Autodesk Inventor part; units mm, degrees
ref_plane "Work Plane1" through (1.525, 0, 0) normal (0, 0, 1) x (1, 0, 0)
ref_plane "YZ Plane" through (0, 0, 0) normal (1, 0, 0) x (0, 1, 0)
ref_plane "XZ Plane" through (0, 0, 0) normal (0, 1, 0) x (-1, 0, 0)
sketch "Sketch1" plane through (0, 0, 0) normal (0, 0, 1) x (1, 0, 0)
  line L0 (0, 7.1374) -> (0, 4.7625)
  line L1 (50.8, 4.7625) -> (76.2, 4.7625)
  line L2 (76.2, 4.7625) -> (76.2, 0)
  line L3 (76.2, 0) -> (-0.6351, 0)
  line L4 (-16.0021, 0) -> (91.567, 0)
  line L5 (-0.6351, 0) -> (-0.6351, 7.1374)
  line L6 (-0.6351, 7.1374) -> (0, 7.1374)
  line L7 (50.8, 4.7625) -> (39.6747, 4.7625)
  line L8 (39.6747, 4.7625) -> (0, 4.7625)
  line L9 (0, -1.4275) -> (0, 8.5649)
  dimension "d0" = 76.2
  dimension "d1" = 25.4
  dimension "d2" = 9.525
  dimension "d9" = 0.6351
  dimension "d10" = 14.2748
  dimension "d13" = 11.1253
  dimension "d14" = 9.525
revolve "Body" add sketch "Sketch1" angle 360 about axis through (76.2, 0, 0) along (-1, 0, 0)
sketch "Sketch2" plane through (-0.6351, 0, 0) normal (-1, 0, 0) x (0, 0, 1)
  line L0 (0, 8.2416) -> (7.1374, 4.1208)
  line L1 (7.1374, 4.1208) -> (7.1374, -4.1208)
  line L2 (7.1374, -4.1208) -> (0, -8.2416)
  line L3 (0, -8.2416) -> (-7.1374, -4.1208)
  line L4 (-7.1374, -4.1208) -> (-7.1374, 4.1208)
  line L5 (-7.1374, 4.1208) -> (0, 8.2416)
  point P0 (0, 0)
  point P1 (0, 0)
  dimension "d11" = 14.2748
extrude "Head" add sketch "Sketch2" along normal blind 5.5372
sketch "Sketch4" plane through (0, 0, 0) normal (0, 0, 1) x (1, 0, 0)
  line L0 (-6.1723, 7.1374) -> (-6.1723, 8.2416)
  line L1 (-6.1723, 8.2416) -> (-5.5348, 8.2416)
  line L2 (-5.5348, 8.2416) -> (-6.1723, 7.1374)
  line L3 (-7.2797, 0) -> (0.4723, 0)
  line L4 (-0.6351, 8.2416) -> (-6.1723, 8.2416)
  line L5 (-6.1723, 4.1208) -> (-6.1723, 8.2416)
  dimension "d5" = 30
  dimension "d19" = 14.2748
revolve "Chamfer1" cut sketch "Sketch4" angle 360 about axis through (-10, 0, 0) along (1, 0, 0)
thread "Thread"
chamfer "Chamfer2" distance 0.9738 distance2 0.9739 1 edges at (76.2, -4.7625, 0) measured on face at (76.2, 1.3701, -0.315)
ref_plane "Work Plane1" through (1.525, 0, 0) normal (0, 0, 1) x (1, 0, 0)
equation "\"d0\" = NLG"
equation "\"d1\" = GEL"
equation "\"d2\" = GD"
equation "\"d10\" = SD2"
equation "\"d14\" = BDM"
equation "\"d11\" = SW"
equation "\"d3\" = KOH - SD"
equation "\"d5\" = ANG1"
equation "\"d19\" = SW0"
equation "\"d15\" = GEL"
equation "\"d6\" = -0.5 * SPD + 0.5 * GD"
equation "\"NLG\" = 76.2"
equation "\"GD\" = 9.525"
equation "\"BDM\" = 9.525"
equation "\"KOH\" = 6.1722"
equation "\"GEL\" = 25.4"
equation "\"SW\" = 14.2748"
equation "\"SW0\" = SW"
equation "\"SPD\" = GD1"
equation "\"SD2\" = SW"
equation "\"SD\" = 0.635"
equation "\"ANG1\" = 30deg"
equation "\"GAL\" = 11.1252"
equation "\"GUL\" = 0.97384"
equation "\"RR\" = 0.381"
equation "\"WFT\" = SD"
equation "\"GD1\" = 7.57733"
equation "\"THREADDIA\" = 9.525"
equation "\"SDH\" = SW"
equation "\"SDHG\" = 39.6748"
equation "\"TOA\" = 30deg"
equation "\"FAWI\" = 45deg"
equation "\"NND\" = 9.525"
equation "\"E0\" = 16.48739"
properties part number "AS 2465 - 3/8 x 3  UNC" material "Steel, Mild"
Check sheet for the modelled part. Datum: model origin and axes. Units: mm. A direction names the side the tool comes from. Round coordinates to 2 decimals unless told otherwise and drop trailing zeros. Write each loop counter-clockwise with the first axis right and the second up, starting at its lowest first coordinate (ties: lowest second). Pieces come first, ordered by that corner, then holes. Notation, with made-up numbers: (-15.5, 74.25) -> (31.5, 74.25) arc R24 ccw to (31.5, 99.25) -> close; hole circle Ø9 at (70, 51). An arc over 180 degrees is marked (long way). Answer as CSV lines item,"result". Start each with the question number.
1) Tool access check on faces 1 (the flat face through (-0.635, -7.5, -0.6)), 2 (the cylindrical face through (-0.31, -7.13, 0.31)), 3 (the flat face through (-0.635, 7.5, -0.6)). Record the directions out of +Z, -Z, +X, -X, +Y, -Y that give a thin tool (end or side, any length) a straight path to the whole face; none if there is none.
2) Section check A-A on x = 65. Enter the section's corners in (y, z) (1 decimal), and give its area (3 significant figures).
3) Material ranges on line 1 (Z direction, x = 58, y = 0); line 2 (X direction, y = -3.5, z = 4); line 3 (Y direction, x = 55, z = -2.5), recorded low to high. Write a range as from..to.
4) Go/stop test with flat-tipped pins: P1, Ø4, axis at x = 16, z = 1.5, coming from the -Y side; P2, Ø1.5, axis at x = 16, y = 1, coming from the -Z side; P3, Ø2, axis at x = 9.5, z = -4.5, coming from the +Y side. Record where each tip stops, or that it passes through.
Found:
1,face 1,"+X, -Y"
1,face 2,"+X"
1,face 3,"+X, +Y"
2,outline,"circle Ø9.5 at (0, 0)"
2,area,"71.3 mm^2"
3,line 1,"z = -4.76..4.76"
3,line 2,"x = -6.17..0"
3,line 3,"y = -4.05..4.05"
4,P1,"stops at y = -4.76"
4,P2,"stops at z = -4.76"
4,P3,"stops at y = 3.23"
